Part print with two shaded views. Sizes in mm from the minimum x, y, z corner. A direction names the side the tool comes from. Give positions to 0.01 mm unless a question says otherwise; leave off trailing zeros. Order: outer loops, then holes, each group sorted by start corner. A loop starts at its lowest first (then second) coordinate and runs counter-clockwise, first axis right, second up. Notation, with made-up numbers: (7.5, -3.5) - (41.5, -3.5) arc R26 cw to (41.5, 23.5) - close; hole circle Ø9 at (40, 67). An arc over 180 degrees is marked (long way). Return JSON: item names as keys, results as strings. Group by question number.
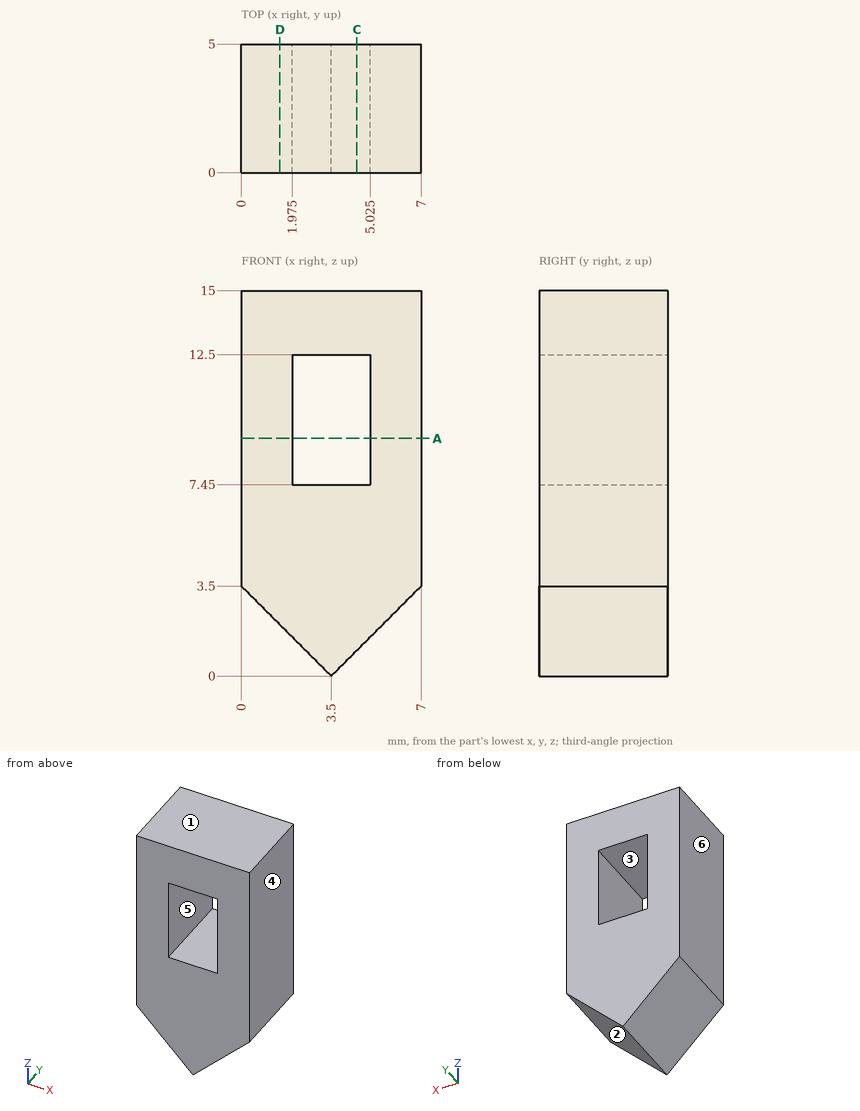
(1) Drop a flat-ended pin along its axis: pin 1 Ø3 at (x, y) = (3, 1.5) entering from -Z. Give the stop position or say it passes through.
(2) Slice it at D-D (x = 1.5). Give the cut face in (y, z), and give its area (3 significant figures).
(3) 3-axis set-ups, long thin cutter, end or side, ignore diameter. For the marked faces 5 and 6: which of +Z, -Z, +X, -X, +Y, -Y reach the whole face in a straight line?
(4) Drill centre lines: L1, parallel to X at y = 2.25, z = 8.5 (3 decimals); L2, parallel to Z at x = 3.75, y = 4.8; L3, parallel to Z at x = 2.75, y = 2.3. Where is each one in solid material? Low to high.
(5) Slice it at C-C (x = 4.5). Give the cut face in (y, z).
(6) Pull direction Z, two halves, no side cores. Call the marked faces 1, 2, 3 and 4: released by +Z, released by -Z, zero draft, split by the parting line, or undercut.
(7) Slice it at A-A (z = 9.25). Give the cut face in (x, y) (3 decimals).
Result set:
{
 "1": {"pin 1": "stops at z = 0"},
 "2": {"outline": "(0, 2) - (5, 2) - (5, 15) - (0, 15) - close", "area": "65.0 mm²"},
 "3": {"face 5": "+Y, -Y", "face 6": "+Z, -Z, -X, +Y, -Y"},
 "4": {"L1": "x = 0 to 1.975, 5.025 to 7", "L2": "z = 0.25 to 7.45, 12.5 to 15", "L3": "z = 0.75 to 7.45, 12.5 to 15"},
 "5": {"outline": "(0, 1) - (5, 1) - (5, 7.45) - (0, 7.45) - close; (0, 12.5) - (5, 12.5) - (5, 15) - (0, 15) - close"},
 "6": {"face 1": "released by +Z", "face 2": "released by -Z", "face 3": "undercut", "face 4": "zero draft"},
 "7": {"outline": "(0, 0) - (1.975, 0) - (1.975, 5) - (0, 5) - close; (5.025, 0) - (7, 0) - (7, 5) - (5.025, 5) - close"}
}
